Check sheet for the modelled part. Datum: model origin and axes. Units: mm. A direction names the side the tool comes from. Coordinates: 2 decimals unless noted, no trailing zeros. Loops run counter-clockwise (first coordinate to the right, second up) from the corner with the lowest first, then second, coordinate; pieces in that order, holes last. Notation, with made-up numbers: M -15,-1.5 L 44,-1.5 A23 ccw 44,11.5 Z; hole C 6,35 d3. An arc over 180 degrees is marked long. Use CSV: the item, a comma, the result in double quotes. Start each with the question number.
(1) Section check D-D on y = 43.25. Give the number of separate pieces and of enclosed holes in the cut face, and give its area (3 significant figures).
(2) Section check B-B on x = 66. Record the cut outline in (y, z), and give its area (3 significant figures).
(3) Section check A-A on z = 15.5. Record the cut outline in (x, y), and give its area (3 significant figures).
(4) Set-up check for faces 1 (the flat face through (135, 43, 25)), 2 (the flat face through (117, 44, 4)), 3 (the flat face through (72, 42, 27)), 4 (the flat face through (47, 43, 47)), 5 (the flat face through (37.5, 44, 23.1)): record each of +Z, -Z, +X, -X, +Y, -Y from which the full face is reachable in a straight line by a thin tool's end or side.
(5) Section check C-C on x = 111. Record the cut outline in (y, z).
(6) Draft check along Z on faces 6 (the flat face through (72, 45, 23)), 7 (the flat face through (37, 44, 50)), 8 (the flat face through (86, 44, 44)). Enter one of: pulls with the +Z half, pulls with the -Z half, needs draft (parallel to the pull), parting line crosses it, or undercut.
(7) Scan lines: line 1 (Z direction, x = 108, y = 44.3); line 2 (X direction, y = 44.45, z = 28); line 3 (Z direction, x = 91, y = 43.25). Record each from-to range of solid material in increasing order.
from build123d import *

# Parameters (mm, degrees)
BOX248_W     = 27.6
BOX248_H     = 2
BOX248_DEPTH = 40.2
BOX249_W     = 27.6
BOX249_H     = 1
BOX249_DEPTH = 32
BOX250_W     = 16
BOX250_H     = 3
BOX250_DEPTH = 8
BOX252_W     = 29.6
BOX252_H     = 1
BOX252_DEPTH = 37.2
BOX251_W     = 31.8
BOX251_H     = 2
BOX251_DEPTH = 39.4
BOX253_W     = 11
BOX253_H     = 3
BOX253_DEPTH = 8
BOX254_W     = 26.8
BOX254_H     = 2
BOX254_DEPTH = 35.9
BOX255_W     = 24.8
BOX255_H     = 1
BOX255_DEPTH = 34.9
BOX263_W     = 24.4
BOX263_H     = 3
BOX263_DEPTH = 24.4
BOX270_W     = 20.7
BOX270_H     = 8.9
BOX270_DEPTH = 2.7
BOX261_W     = 24.4
BOX261_H     = 1
BOX261_DEPTH = 13.8
BOX262_W     = 26.6
BOX262_H     = 1
BOX262_DEPTH = 3
BOX260_W     = 26.6
BOX260_H     = 2
BOX260_DEPTH = 16
BOX247_W     = 135
BOX247_H     = 3
BOX247_DEPTH = 50


with BuildPart() as cut_out_cam_large:
    # Box248 → Box248 (new body)
    with BuildSketch(Plane(origin=(5, 42, 5), x_dir=(1, 0, 0), z_dir=(0, 0, 1))):
        with Locations((13.8, 1)):
            Rectangle(BOX248_W, BOX248_H)
    extrude(amount=BOX248_DEPTH)


with BuildPart() as cut_out_cam_small:
    # Box249 → Box249 (new body)
    with BuildSketch(Plane(origin=(5, 44, 10), x_dir=(1, 0, 0), z_dir=(0, 0, 1))):
        with Locations((13.8, 0.5)):
            Rectangle(BOX249_W, BOX249_H)
    extrude(amount=BOX249_DEPTH)


with BuildPart() as cut_out_esp32cam:
    # Box250 → Box250 (new body)
    with BuildSketch(Plane(origin=(11, 42, 42), x_dir=(1, 0, 0), z_dir=(0, 0, 1))):
        with Locations((8, 1.5)):
            Rectangle(BOX250_W, BOX250_H)
    extrude(amount=BOX250_DEPTH)

    # Fusion: union cut-out cam large, cut-out cam small
    add(cut_out_cam_large.part)
    add(cut_out_cam_small.part)


with BuildPart() as cube225:
    # Box252 → Box252 (new body)
    with BuildSketch(Plane(origin=(38, 44, 6), x_dir=(1, 0, 0), z_dir=(0, 0, 1))):
        with Locations((14.8, 0.5)):
            Rectangle(BOX252_W, BOX252_H)
    extrude(amount=BOX252_DEPTH)


with BuildPart() as cube224:
    # Box251 → Box251 (new body)
    with BuildSketch(Plane(origin=(37, 42, 5), x_dir=(1, 0, 0), z_dir=(0, 0, 1))):
        with Locations((15.9, 1)):
            Rectangle(BOX251_W, BOX251_H)
    extrude(amount=BOX251_DEPTH)


with BuildPart() as cut_out_esp32:
    # Box253 → Box253 (new body)
    with BuildSketch(Plane(origin=(47, 42, 42), x_dir=(1, 0, 0), z_dir=(0, 0, 1))):
        with Locations((5.5, 1.5)):
            Rectangle(BOX253_W, BOX253_H)
    extrude(amount=BOX253_DEPTH)

    # Fusion066: union Cube225, Cube224
    add(cube225.part)
    add(cube224.part)


with BuildPart() as cube227:
    # Box254 → Box254 (new body)
    with BuildSketch(Plane(origin=(73, 42, 5), x_dir=(1, 0, 0), z_dir=(0, 0, 1))):
        with Locations((13.4, 1)):
            Rectangle(BOX254_W, BOX254_H)
    extrude(amount=BOX254_DEPTH)


with BuildPart() as obj1:
    # Box255 → Box255 (new body)
    with BuildSketch(Plane(origin=(74, 44, 6), x_dir=(1, 0, 0), z_dir=(0, 0, 1))):
        with Locations((12.4, 0.5)):
            Rectangle(BOX255_W, BOX255_H)
    extrude(amount=BOX255_DEPTH)

    # Fusion067: union Cube227
    add(cube227.part)


with BuildPart() as cut_out_gps_antenna:
    # Box263 → Box263 (new body)
    with BuildSketch(Plane(origin=(105, 42, 4), x_dir=(1, 0, 0), z_dir=(0, 0, 1))):
        with Locations((12.2, 1.5)):
            Rectangle(BOX263_W, BOX263_H)
    extrude(amount=BOX263_DEPTH)


with BuildPart() as cut_out_header:
    # Box270 → Box270 (new body)
    with BuildSketch(Plane(origin=(76, 36.5, 44), x_dir=(1, 0, 0), z_dir=(0, 0, 1))):
        with Locations((10.35, 4.45)):
            Rectangle(BOX270_W, BOX270_H)
    extrude(amount=BOX270_DEPTH)


with BuildPart() as cube234:
    # Box261 → Box261 (new body)
    with BuildSketch(Plane(origin=(103, 44, 30), x_dir=(1, 0, 0), z_dir=(0, 0, 1))):
        with Locations((12.2, 0.5)):
            Rectangle(BOX261_W, BOX261_H)
    extrude(amount=BOX261_DEPTH)


with BuildPart() as cube235:
    # Box262 → Box262 (new body)
    with BuildSketch(Plane(origin=(102, 44, 42), x_dir=(1, 0, 0), z_dir=(0, 0, 1))):
        with Locations((13.3, 0.5)):
            Rectangle(BOX262_W, BOX262_H)
    extrude(amount=BOX262_DEPTH)


with BuildPart() as cut_outs:
    # Box260 → Box260 (new body)
    with BuildSketch(Plane(origin=(102, 42, 29), x_dir=(1, 0, 0), z_dir=(0, 0, 1))):
        with Locations((13.3, 1)):
            Rectangle(BOX260_W, BOX260_H)
    extrude(amount=BOX260_DEPTH)

    # Fusion070: union Cube234, Cube235
    add(cube234.part)
    add(cube235.part)


with BuildPart() as cut_outs_1:
    # Fusion070 placement: moved
    add(cut_outs.part.moved(Location((2, 0, 2))))

    # Fusion071: union Cut-out ESP32CAM, Cut-out ESP32, obj1, Cut-out GPS antenna, Cut-out header
    add(cut_out_esp32cam.part)
    add(cut_out_esp32.part)
    add(obj1.part)
    add(cut_out_gps_antenna.part)
    add(cut_out_header.part)


with BuildPart() as plate:
    # Box247 → Box247 (new body)
    with BuildSketch(Plane(origin=(0, 42, 0), x_dir=(1, 0, 0), z_dir=(0, 0, 1))):
        with Locations((67.5, 1.5)):
            Rectangle(BOX247_W, BOX247_H)
    extrude(amount=BOX247_DEPTH)

    # Cut197: cut  Cut-outs
    add(cut_outs_1.part, mode=Mode.SUBTRACT)


solid = plate.part
Outcome:
1,separate pieces,"1"
1,enclosed holes,"4"
1,area,"2,210 mm²"
2,outline,"M 42,0 L 45,0 L 45,6 L 44,6 L 44,5 L 42,5 Z; M 42,44.4 L 44,44.4 L 44,43.2 L 45,43.2 L 45,50 L 42,50 Z"
2,area,"34.0 mm²"
3,outline,"M 0,42 L 5,42 L 5,45 L 0,45 Z; M 32.6,42 L 37,42 L 37,44 L 38,44 L 38,45 L 32.6,45 Z; M 67.6,44 L 68.8,44 L 68.8,42 L 73,42 L 73,44 L 74,44 L 74,45 L 67.6,45 Z; M 98.8,44 L 99.8,44 L 99.8,42 L 105,42 L 105,45 L 98.8,45 Z; M 129.4,42 L 135,42 L 135,45 L 129.4,45 Z"
3,area,"77.4 mm²"
4,face 1,"+Z, -Z, +X, +Y, -Y"
4,face 2,"+Y, -Y"
4,face 3,"+Z, -Z, +X, -X, -Y"
4,face 4,"+Z, +Y, -Y"
4,face 5,"-Y"
5,outline,"M 42,0 L 45,0 L 45,4 L 42,4 Z; M 42,28.4 L 45,28.4 L 45,32 L 44,32 L 44,31 L 42,31 Z; M 42,47 L 45,47 L 45,50 L 42,50 Z"
6,face 6,"needs draft"
6,face 7,"pulls with the +Z half"
6,face 8,"undercut"
7,line 1,"z = 0 to 4, 28.4 to 32, 47 to 50"
7,line 2,"x = 0 to 5, 32.6 to 38, 67.6 to 74, 98.8 to 105, 129.4 to 135"
7,line 3,"z = 0 to 5, 40.9 to 44, 46.7 to 50"
